Autodesk Inventor part; units mm, degrees
ref_plane "YZ Plane" through (0, 0, 0) normal (1, 0, 0) x (0, 1, 0)
ref_plane "XZ Plane" through (0, 0, 0) normal (0, 1, 0) x (-1, 0, 0)
ref_plane "XY Plane" through (0, 0, 0) normal (0, 0, 1) x (1, 0, 0)
sketch "草图1" plane through (0, 0, 0) normal (0, 0, 1) x (1, 0, 0)
  line L0 (0, 0) -> (57, 0)
  line L1 (57, 0) -> (75, 0)
  line L2 (75, 0) -> (75, 20)
  line L3 (0, 0) -> (0, 140)
  line L4 (0, 140) -> (55, 140)
  line L5 (0, 140) -> (40, 140)
  line L6 (40, 140) -> (40, 120)
  line L7 (40, 120) -> (32.5, 120)
  line L8 (32.5, 120) -> (32.5, 60)
  line L9 (32.5, 60) -> (40, 60)
  line L10 (57, 0) -> (57, 3)
  line L11 (57, 3) -> (0, 3)
  line L12 (0, 3) -> (43, 3)
  line L13 (43, 3) -> (40, 60)
  line L14 (75, 20) -> (0, 20)
  line L15 (0, 20) -> (60, 20)
  line L16 (60, 20) -> (55, 140)
  dimension "d0" = 57
  dimension "d1" = 18
  dimension "d2" = 20
  dimension "d3" = 140
  dimension "d4" = 55
  dimension "d5" = 40
  dimension "d6" = 20
  dimension "d7" = 7.5
  dimension "d10" = 7.5
  dimension "d11" = 3
  dimension "d12" = 43
  dimension "d13" = 60
revolve "旋转1" add sketch "草图1" angle 360 about axis through (0, 0, 0) along (0, 1, 0) contours L10 L11 L13 L14 L2 L1 | L13 L9 L8 L7 L6 L4 L16 L14
fillet "圆角1" radius 2 1 edges at (-75, 20, 0)
fillet "圆角2" radius 2 1 edges at (-60, 20, 0)
fillet "圆角3" radius 2 1 edges at (-55, 140, 0)
sketch "草图2" plane through (0, 140, 0) normal (0, 1, 0) x (1, 0, 0)
  circle A0 centre (0, 0) radius 40
  point P0 (0, 40)
hole "孔1" at (0, 140, -40) direction (0, -1, 0) diameter 8.376 depth 17
properties part number "底座"
Check sheet for the modelled part. Datum: model origin and axes. Units: mm. A direction names the side the tool comes from. Give positions to 0.01 mm unless a question says otherwise; leave off trailing zeros. Write each loop counter-clockwise with the first axis right and the second up, starting at its lowest first coordinate (ties: lowest second). Pieces come first, ordered by that corner, then holes.
Item 1: Cross-section at C-C (y = 96.5). Enter the section's corners in (x, z) (1 decimal).
Item 2: Gauge pin test, flat ends, axial feed: pin 1 (1.5 mm diameter, centred on y = 88.5, z = 29, fed in from +X); pin 2 (24 mm diameter, centred on x = 10.5, z = -12, fed in from -Y); pin 3 (3 mm diameter, centred on x = -41.5, z = 60, fed in from +Y); pin 4 (1 mm diameter, centred on x = -20, y = 46.5, fed in from -Z). Record the tip position at first contact, or that the pin passes through.
Item 3: Access from +Z, -Z, +X, -X, +Y, -Y to the whole of each face (thin tool, end or side, straight path). Record for faces 1 (the face through (-8, 140, -40)), 2 (the face through (0, 60, -33)), 3 (the face through (-8.67, 129.86, -39.05)).
Item 4: Draft check along X on faces 4 (the face through (8.2, 3, -42.5)), 5 (the face through (-33, 20, 54)), 6 (the face through (54.877, 79.187, 17.282)). Enter one of: released by +X, released by -X, zero draft, split by the parting line, or undercut.
Item 5: Cross-section at D-D (y = 66). Enter the section's corners in (x, z).
Item 6: Scan lines: L1, parallel to X at y = 1.8, z = 0; L2, parallel to Z at x = 10, y = 28. Record each from-to range of solid material in increasing order.
Report:
1. outline: circle Ø113.6 at (0, 0); hole circle Ø65 at (0, 0)
2. pin 1: stops at x = 49.68
2. pin 2: passes through
2. pin 3: stops at y = 20
2. pin 4: stops at z = -55.58
3. face 1: +Z, -Z, +X, -X, +Y
3. face 2: -Y
3. face 3: +Y
4. face 4: undercut
4. face 5: zero draft
4. face 6: split by the parting line
5. outline: circle Ø116.17 at (0, 0); hole circle Ø65 at (0, 0)
6. L1: x = -75 to -57, 57 to 75
6. L2: z = -58.82 to -40.47, 40.47 to 58.82
